Geometry check sheet. Reference: the model listing, model coordinates, mm. Face numbers are marked on the shaded views. A direction names the side the tool comes from. Coordinates: 2 decimals unless noted, no trailing zeros. Write each loop counter-clockwise with the first axis right and the second up, starting at its lowest first coordinate (ties: lowest second). Pieces come first, ordered by that corner, then holes.
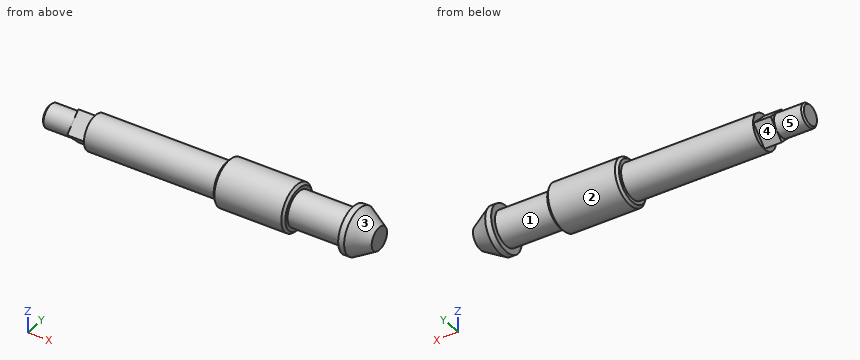
from build123d import *

# Parameters (mm, degrees)
CHAMFER_1_SIZE      = 0.828
SKETCH_2_R          = 6
SKETCH_2_R_2        = 4
CUT_EXTRUDE_1_DEPTH = 10
SKETCH_3_R          = 6
CUT_EXTRUDE_2_DEPTH = 6
CHAMFER_2_SIZE      = 0.5545


with BuildPart() as part:
    # Эскиз1 → Повернуть1 (revolve)
    with BuildSketch(Plane.XY):
        Polygon((0, 0), (0, 4), (-6.92820323, 8), (-9, 8), (-9, 6), (-28, 6), (-28, 8), (-53, 8), (-53, 6), (-115, 6), (-115, 0), align=None)
    revolve(axis=Axis((0, 0, 0), (-1, 0, 0)))

    # Фаска1
    chamfer_1_edges = [part.edges().sort_by_distance(p)[0] for p in [
        (-53, -8, 0),
        (-28, -8, 0),
    ]]
    chamfer(chamfer_1_edges, length=CHAMFER_1_SIZE)

    # Эскиз2 → Вырез-Вытянуть1 (cut)
    with BuildSketch(Plane.ZY.offset(115)):
        Circle(SKETCH_2_R)
        Circle(SKETCH_2_R_2, mode=Mode.SUBTRACT)
    extrude(amount=-CUT_EXTRUDE_1_DEPTH, mode=Mode.SUBTRACT)

    # Эскиз3 → Вырез-Вытянуть2 (cut)
    with BuildSketch(Plane.ZY.offset(105)):
        Circle(SKETCH_3_R)
        Polygon((0, 5.798275606), (-5.798275606, 0), (0, -5.798275606), (5.798275606, 0), align=None, mode=Mode.SUBTRACT)
    extrude(amount=-CUT_EXTRUDE_2_DEPTH, mode=Mode.SUBTRACT)

    # Фаска2
    chamfer_2_edges = [part.edges().sort_by_distance(p)[0] for p in [
        (-115, 0, -4),
    ]]
    chamfer(chamfer_2_edges, length=CHAMFER_2_SIZE)


solid = part.part
1. Thickness scan on line 1 along X through (y, z) = (-0.75, 6.5); line 2 along X through (y, z) = (7, -2.25); line 3 along X through (y, z) = (2.5, -5). Record the ranges inside material, lowest first.
Computed values:
line 1: x = -53 to -28, -9 to -4.4
line 2: x = -52.82 to -28.18, -9 to -5.81
line 3: x = -99 to -2.75
2. Access from +Z, -Z, +X, -X, +Y, -Y to the whole of each face (thin tool, end or side, straight path). Record for the marked faces 4 and 5.
Computed values:
face 4: -Z, -X, +Y
face 5: -X
3. Sectioned sample at A-A, the plane x = -92. Record the boundary of the cut face in (y, z), and give its area (3 significant figures).
Computed values:
outline: circle Ø12 at (0, 0)
area: 113 mm2
4. Draft check along X on the marked faces 1, 2 and 3. Enter one of: released by +X, released by -X, zero draft, split by the parting line, or undercut.
Computed values:
face 1: undercut
face 2: zero draft
face 3: released by +X
5. Gauge pin test, flat ends, axial feed: pin 1 Ø8 at (x, z) = (-42, -5.5) entering from +Y; pin 2 Ø1 at (x, z) = (-40, -4.5) entering from +Y; pin 3 Ø1 at (x, y) = (-87.5, -4) entering from +Z. Record the tip position at first contact, or that the pin passes through.
Computed values:
pin 1: stops at y = 7.86
pin 2: stops at y = 6.93
pin 3: stops at z = 4.87
6. Sectioned sample at B-B, the plane x = -35.5. Record the boundary of the cut face in (y, z).
Computed values:
outline: circle Ø16 at (0, 0)
